The model under review builds one solid part; all positions refer to its coordinate system, in mm. Face numbers are marked on the shaded views. A direction names the side the tool comes from. Round coordinates to 2 decimals unless told otherwise and drop trailing zeros. Order: outer loops, then holes, each group sorted by start corner. A loop starts at its lowest first (then second) coordinate and runs counter-clockwise, first axis right, second up. Notation, with made-up numbers: M 40,67.5 L 45,67.5 A18 ccw 45,81.5 Z; hole C -20.75,-28.75 d1. An arc over 180 degrees is marked long. Answer as a JSON object with one key per item and string values. Group by question number.
1. Clearance check with flat-ended pins moving along their axes: P1, Ø4, axis at x = -1, z = 25, coming from the -Y side; P2, Ø1.5, axis at x = 0, y = -0.5, coming from the -Z side; P3, Ø2, axis at x = -2.5, z = 25.5, coming from the +Y side. State where each tip first meets the part, or that it passes through.
2. To check wall thickness, follow probe 1 along Z at (x, y) = (-1.5, 0); probe 2 along Z at (x, y) = (-0.25, -2.5); probe 3 along Y at (x, z) = (0.75, 11). State the ranges of each line that lie inside material, in increasing order. Write a range as [from, to].
3. Add section C-C on x = -2.5. State the section outline as (y, z) points.
4. Add section B-B on z = 31.5. State the section outline as (x, y) points, and give its area (3 significant figures).
5. Machinability: for the marked faces 1 and 2, which of the approach directions +Z, -Z, +X, -X, +Y, -Y give a long, thin tool a straight path to every point of the face, cutting with its end or side? Answer none if there is none.
6. Add section A-A on x = 0. State the section outline as (y, z) points, and give its area (3 significant figures).
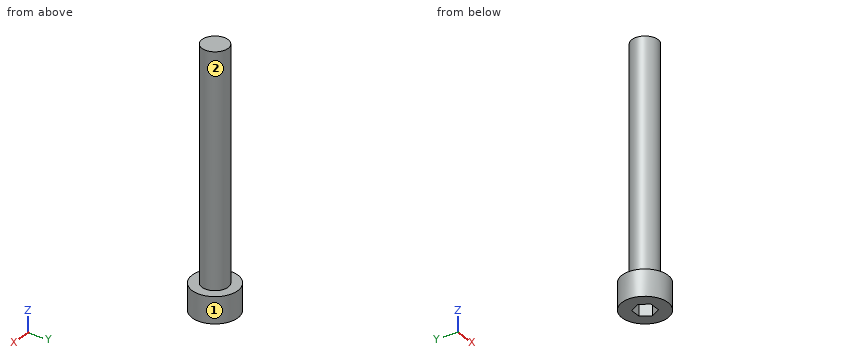
Solid Edge part; units mm, degrees
sketch "Sketch1" plane through (0, 0, 0) normal (0, 0, 1) x (1, 0, 0)
  circle A0 centre (0, 0) radius 3.5
extrude "Protrusion1" add sketch "Sketch1" along normal blind 4
sketch "Sketch2" plane through (0, 0, 0) normal (0, 0, -1) x (1, 0, 0)
  line L0 (0.85, 1.4722) -> (1.7, 0)
  line L1 (1.7, 0) -> (0.85, -1.4722)
  line L2 (0.85, -1.4722) -> (-0.85, -1.4722)
  line L3 (-0.85, -1.4722) -> (-1.7, 0)
  line L4 (-1.7, 0) -> (-0.85, 1.4722)
  line L5 (-0.85, 1.4722) -> (0.85, 1.4722)
extrude "ExtrudedCutout_1" cut sketch "Sketch2" against normal blind 2.4
sketch "Sketch3" plane through (0, 0, 4) normal (0, 0, 1) x (-1, 0, 0)
  circle A0 centre (0, 0) radius 2
extrude "ExtrudedProtrusion_2" add sketch "Sketch3" along normal blind 35
cosmetic_thread "Thread_2" thread depth 20
Recorded:
{
 "1": {"P1": "stops at y = -2", "P2": "stops at z = 2.4", "P3": "stops at y = 1.32"},
 "2": {"probe 1": "z = [2.4, 39]", "probe 2": "z = [0, 4]", "probe 3": "y = [-1.85, 1.85]"},
 "3": {"outline": "M -2.45,0 L 2.45,0 L 2.45,4 L -2.45,4 Z"},
 "4": {"outline": "C 0,0 d4", "area": "12.6 mm²"},
 "5": {"face 1": "+Z, -Z", "face 2": "+Z"},
 "6": {"outline": "M -3.5,0 L -1.47,0 L -1.47,2.4 L 1.47,2.4 L 1.47,0 L 3.5,0 L 3.5,4 L 2,4 L 2,39 L -2,39 L -2,4 L -3.5,4 Z", "area": "161 mm²"}
}
